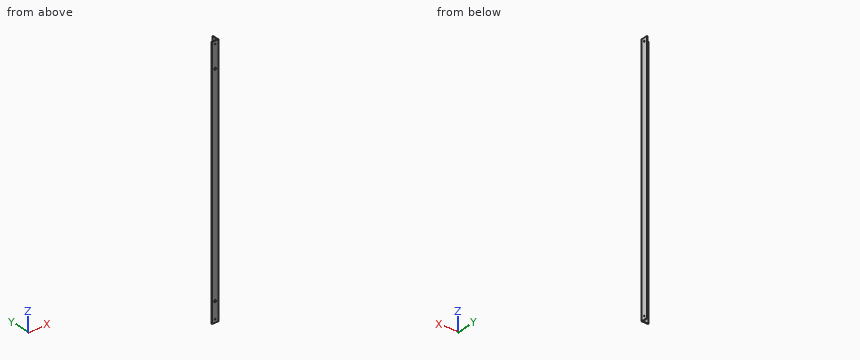
```python
from build123d import *

# Parameters (mm, degrees)
BOSS_EXTRUDE1_DEPTH = 762
SKETCH2_R           = 1.5875
SKETCH2_R_2         = 3.175
CUT_EXTRUDE2_DEPTH  = 2.794
SKETCH4_R           = 1.5875
CUT_EXTRUDE3_DEPTH  = 8.89
SKETCH5_W           = 19.05
SKETCH5_H           = 19.05
CUT_EXTRUDE4_DEPTH  = 764.189696275


with BuildPart() as part:
    # Sketch1 → Boss-Extrude1 (new body)
    with BuildSketch(Plane.XY):
        Polygon((0, 0), (0, 19.05), (1.5875, 19.05), (1.5875, 1.5875), (19.05, 1.5875), (19.05, 0), align=None)
    boss_extrude1 = extrude(amount=-BOSS_EXTRUDE1_DEPTH)

    # Sketch2 → Cut-Extrude2 (cut)
    with BuildSketch(Plane(origin=(0, 1.5875, 0), x_dir=(1, 0, 0), z_dir=(0, 1, 0))):
        with Locations(Location((9.525, 9.525, 0), (0, 0, 270))):
            Circle(SKETCH2_R)
        with Locations(Location((9.525, 752.475, 0), (0, 0, 270))):
            Circle(SKETCH2_R)
        with Locations(Location((9.525, 76.2, 0), (0, 0, 270))):
            Circle(SKETCH2_R_2)
        with Locations(Location((9.525, 703.58, 0), (0, 0, 270))):
            Circle(SKETCH2_R_2)
    cut_extrude2 = extrude(amount=-CUT_EXTRUDE2_DEPTH, mode=Mode.SUBTRACT)

    # Sketch4 → Cut-Extrude3 (cut)
    with BuildSketch(Plane(origin=(1.5875, 0, 0), x_dir=(0, 0, -1), z_dir=(1, 0, 0))):
        with Locations((9.525, 9.525)):
            Circle(SKETCH4_R)
        with Locations((752.475, 9.525)):
            Circle(SKETCH4_R)
    cut_extrude3 = extrude(amount=-CUT_EXTRUDE3_DEPTH, mode=Mode.SUBTRACT)

    # Mirror1: Boss-Extrude1, Cut-Extrude2, Cut-Extrude3 across plane
    add(boss_extrude1.mirror(Plane(origin=(19.05, 0, -762), x_dir=(0, 0, 1), z_dir=(1, 0, 0))))
    add(cut_extrude2.mirror(Plane(origin=(19.05, 0, -762), x_dir=(0, 0, 1), z_dir=(1, 0, 0))), mode=Mode.SUBTRACT)
    add(cut_extrude3.mirror(Plane(origin=(19.05, 0, -762), x_dir=(0, 0, 1), z_dir=(1, 0, 0))), mode=Mode.SUBTRACT)

    # Sketch5 → Cut-Extrude4 (cut, through all)
    with BuildSketch(Plane.XY):
        with Locations((9.525, 9.525)):
            Rectangle(SKETCH5_W, SKETCH5_H)
    extrude(amount=-CUT_EXTRUDE4_DEPTH, mode=Mode.SUBTRACT)


solid = part.part
```
Geometry: final body of the model. Coordinates: model frame, mm. Round coordinates to 2 decimals unless told otherwise and drop trailing zeros. Write each loop counter-clockwise with the first axis right and the second up, starting at its lowest first coordinate (ties: lowest second). Pieces come first, ordered by that corner, then holes. Notation, with made-up numbers: M -26,-1.75 L 24,-1.75 A11 ccw 24,8.25 Z; hole C 26,42.25 d7. An arc over 180 degrees is marked long. Answer in a Markdown table with one row per item. Add a question column.
(1) Cut plane B-B, the plane y = 15.5. Return the cut outline in (x, z), then the cut area to 3 significant figures.
(2) Ray query, L1, parallel to X at y = 1.15, z = -703.58; L2, parallel to Y at x = 28, z = -215; L3, parallel to X at y = 16.25, z = -236. Return the intervals inside material, ascending.
(3) Cut plane A-A, the plane z = -514.5. Return the cut outline in (x, y), then the cut area to 3 significant figures.
(4) Contact query for flat-ended pins moving along their axis: pin 1 (6 mm diameter, centred on x = 22.5, z = -291, fed in from -Y); pin 2 (5 mm diameter, centred on x = 28.575, z = -76.2, fed in from -Y). Output: stop coordinate, or through.
Established:
| question | item | result |
|---|---|---|
| 1 | outline | M 36.51,-762 L 38.1,-762 L 38.1,0 L 36.51,0 Z |
| 1 | area | 1,210 mm² |
| 2 | L1 | 19.05 to 25.4, 31.75 to 38.1 |
| 2 | L2 | 0 to 1.59 |
| 2 | L3 | 36.51 to 38.1 |
| 3 | outline | M 19.05,0 L 38.1,0 L 38.1,19.05 L 36.51,19.05 L 36.51,1.59 L 19.05,1.59 Z |
| 3 | area | 58.0 mm² |
| 4 | pin 1 | y = 0 |
| 4 | pin 2 | through |
